Geometry: final body of the model. Coordinates: model frame, mm. Face numbers are marked on the shaded views. Round coordinates to 2 decimals unless told otherwise and drop trailing zeros. Loops run counter-clockwise (first coordinate to the right, second up) from the corner with the lowest first, then second, coordinate; pieces in that order, holes last. Notation, with made-up numbers: (-11, 66) - (1, 66) arc R5 cw to (1, 70) - close; hole circle Ø4 at (51.25, 77). An arc over 180 degrees is marked (long way). Answer in a Markdown table with one row per item. Add a question column.
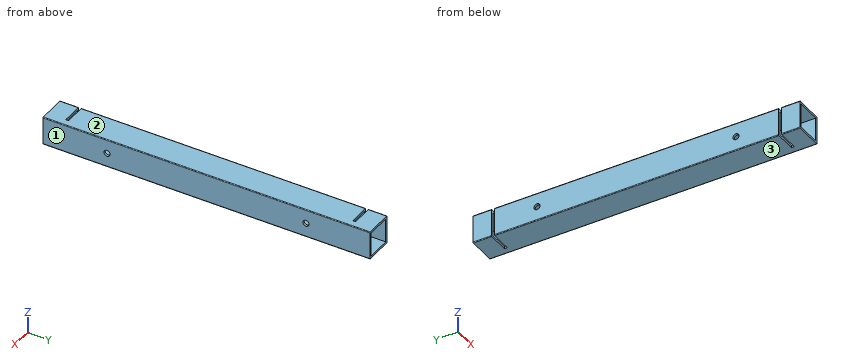
from build123d import *

# Parameters (mm, degrees)
SKETCH1_W           = 17
SKETCH1_H           = 17
BOSS_EXTRUDE1_DEPTH = 230
SKETCH2_W           = 20
SKETCH2_H           = 2
CUT_EXTRUDE1_DEPTH  = 15
SKETCH3_R           = 2.15
CUT_EXTRUDE2_DEPTH  = 232.732604525


with BuildPart() as part:
    # Sketch1 → Boss-Extrude1 (new body)
    with BuildSketch(Plane(origin=(0, 0, 0), x_dir=(1, 0, 0), z_dir=(0, 1, 0))):
        with BuildLine():
            Line((0.5, 0), (19.5, 0))
            ThreePointArc((19.5, 0), (19.853553391, 0.146446609), (20, 0.5))
            Line((20, 0.5), (20, 19.5))
            ThreePointArc((20, 19.5), (19.853553391, 19.853553391), (19.5, 20))
            Line((19.5, 20), (0.5, 20))
            ThreePointArc((0.5, 20), (0.146446609, 19.853553391), (0, 19.5))
            Line((0, 19.5), (0, 0.5))
            ThreePointArc((0, 0.5), (0.146446609, 0.146446609), (0.5, 0))
        make_face()
        with Locations((10, 10)):
            Rectangle(SKETCH1_W, SKETCH1_H, mode=Mode.SUBTRACT)
    extrude(amount=BOSS_EXTRUDE1_DEPTH)

    # Sketch2 → Cut-Extrude1 (cut)
    with BuildSketch(Plane.ZY):
        with Locations((-10, 14)):
            Rectangle(SKETCH2_W, SKETCH2_H)
        with Locations((-10, 216)):
            Rectangle(SKETCH2_W, SKETCH2_H)
    extrude(amount=-CUT_EXTRUDE1_DEPTH, mode=Mode.SUBTRACT)

    # Sketch3 → Cut-Extrude2 (cut, through all)
    with BuildSketch(Plane(origin=(20, 0, 0), x_dir=(0, 0, -1), z_dir=(1, 0, 0))):
        with Locations((10, 185)):
            Circle(SKETCH3_R)
        with Locations(Location((10, 45, 0), (0, 0, 180))):
            Circle(SKETCH3_R)
    extrude(amount=-CUT_EXTRUDE2_DEPTH, mode=Mode.SUBTRACT)


solid = part.part
1) Pull-direction query (Z, two-part tool) for the marked faces 1, 2 and 3; classes: pulls with the +Z half, pulls with the -Z half, needs draft (parallel to the pull), parting line crosses it, or undercut.
2) Material intervals for line 1 along Y through (x, z) = (1, -16.25); line 2 along Y through (x, z) = (0.95, -10); line 3 along Y through (x, z) = (19.35, -10), sorted ascending. Write a range as from..to.
3) Section A-A, the plane z = -10. Give the number of separate pieces and of enclosed holes in the cut face, and give its area (3 significant figures).
4) Contact query for flat-ended pins moving along their axis: pin 1 Ø0.8 at (y, z) = (216, -19.5) entering from -X; pin 2 Ø4 at (y, z) = (45, -10) entering from -X; pin 3 Ø12 at (x, y) = (3, 196) entering from +Z. Output: stop coordinate, or through.
5) Section C-C, the plane y = 185. Return the cut outline in (x, z), and give its area (3 significant figures).
6) Section B-B, the plane x = 6.75. Return the cut outline in (y, z), and give its area (3 significant figures).
7) Section D-D, the plane y = 160. Return the cut outline in (x, z).
Evaluation:
| question | item | result |
|---|---|---|
| 1 | face 1 | needs draft |
| 1 | face 2 | pulls with the +Z half |
| 1 | face 3 | pulls with the -Z half |
| 2 | line 1 | y = 0..13, 15..215, 217..230 |
| 2 | line 2 | y = 0..13, 15..42.85, 47.15..182.85, 187.15..215, 217..230 |
| 2 | line 3 | y = 0..42.85, 47.15..182.85, 187.15..230 |
| 3 | separate pieces | 8 |
| 3 | enclosed holes | 0 |
| 3 | area | 658 mm² |
| 4 | pin 1 | stops at x = 15 |
| 4 | pin 2 | passes through |
| 4 | pin 3 | stops at z = 0 |
| 5 | outline | (0, -19.5) arc R0.5 ccw to (0.5, -20) - (19.5, -20) arc R0.5 ccw to (20, -19.5) - (20, -12.15) - (18.5, -12.15) - (18.5, -18.5) - (1.5, -18.5) - (1.5, -12.15) - (0, -12.15) - close; (0, -7.85) - (1.5, -7.85) - (1.5, -1.5) - (18.5, -1.5) - (18.5, -7.85) - (20, -7.85) - (20, -0.5) arc R0.5 ccw to (19.5, 0) - (0.5, 0) arc R0.5 ccw to (0, -0.5) - close |
| 5 | area | 97.9 mm² |
| 6 | outline | (0, -20) - (13, -20) - (13, -18.5) - (0, -18.5) - close; (0, -1.5) - (13, -1.5) - (13, 0) - (0, 0) - close; (15, -20) - (215, -20) - (215, -18.5) - (15, -18.5) - close; (15, -1.5) - (215, -1.5) - (215, 0) - (15, 0) - close; (217, -20) - (230, -20) - (230, -18.5) - (217, -18.5) - close; (217, -1.5) - (230, -1.5) - (230, 0) - (217, 0) - close |
| 6 | area | 678 mm² |
| 7 | outline | (0, -19.5) arc R0.5 ccw to (0.5, -20) - (19.5, -20) arc R0.5 ccw to (20, -19.5) - (20, -0.5) arc R0.5 ccw to (19.5, 0) - (0.5, 0) arc R0.5 ccw to (0, -0.5) - close; hole (1.5, -18.5) - (18.5, -18.5) - (18.5, -1.5) - (1.5, -1.5) - close |
